The listing builds one solid part. Answer for the finished solid, in the listing's coordinates (mm). A direction names the side the tool comes from. Give positions to 0.01 mm unless a question says otherwise; leave off trailing zeros. Order: outer loops, then holes, each group sorted by start corner. A loop starts at its lowest first (then second) coordinate and runs counter-clockwise, first axis right, second up. Notation, with made-up numbers: (54.5, 72) - (62.5, 72) arc R23 cw to (62.5, 105) - close; hole circle Ø11 at (46.5, 9.25). An arc over 180 degrees is marked (long way). Write each question's results on one line, items separated by ' | '. Start each with the question number.
1. Find the intervals of material crossed by L1, parallel to X at y = 29, z = 19 (3 decimals); L2, parallel to Y at x = 2, z = 1; L3, parallel to X at y = 25, z = 20, in increasing order.
2. Flat-ended cylindrical pins translate along their axes: pin 1 (2 mm diameter, centred on x = 15.5, z = 27.5, fed in from +Y); pin 2 (10 mm diameter, centred on y = -12.5, z = -4.5, fed in from +X); pin 3 (2 mm diameter, centred on x = -3, y = 62, fed in from +Z). Find the tip coordinate at first contact, or state that the pin passes through.
3. Section A-A (y = 38.1) is taken. Give the vertices of the cut face in (x, z) (3 decimals).
4. Determine the mould class of faces 1 (the face through (-16, 3.175, -5)), 2 (the face through (22.225, 38, 9)), 3 (the face through (-25.4, 39, 18)) for opening direction X: released by +X, released by -X, zero draft, split by the parting line, or undercut.
5. Which of the six approach directions +Z, -Z, +X, -X, +Y, -Y give full straight-line access (tool end or side, diameter ignored) to faces 4 (the face through (-22.225, 38, 9)), 5 (the face through (15.92, -2.77, 14.06)), 6 (the face through (16, 3.175, -5)), 7 (the face through (15.349, -16.724, -11.197))?
from build123d import *

# Parameters (mm, degrees)
BOSS_EXTRUDE1_DEPTH                 = 25.4
SHELL1_T                            = -3.175
SKETCH4_R                           = 12.7
BOSS_EXTRUDE3_DEPTH                 = 19.05
BOSS_EXTRUDE4_DEPTH                 = 19.05
SKETCH6_R                           = 12.7
CUT_EXTRUDE2_DEPTH                  = 12.7
CUT_EXTRUDE3_START                  = 12.7
SKETCH6_2_R                         = 12.7
CUT_EXTRUDE3_DEPTH                  = 12.7
CUT_EXTRUDE4_REACH                  = 98.093
SKETCH7_R                           = 3.175
BOSS_EXTRUDE5_REACH                 = 98.093
CUT_EXTRUDE5_DEPTH                  = 12.7
BOSS_EXTRUDE6_DEPTH                 = 25.4
FILLET2_R                           = 12.7
CUT_EXTRUDE6_REACH                  = 109.812
CUT_EXTRUDE6_END_RADIUS             = 3.175
SKETCH12_R                          = 1.7526
CUT_EXTRUDE6_DIRECTION_2_REACH      = 109.812
CUT_EXTRUDE6_DIRECTION_2_END_RADIUS = 12.7
CUT_EXTRUDE7_DEPTH                  = 108.812149615


with BuildPart() as part:
    # Sketch2 → Boss-Extrude1 (new, symmetric)
    with BuildSketch(Plane(origin=(0, 0, 0), x_dir=(0, 0, -1), z_dir=(1, 0, 0))):
        with BuildLine():
            Line((0, 0), (0, 76.2))
            ThreePointArc((0, 76.2), (-38.1, 38.1), (0, 0))
        make_face()
    extrude(amount=BOSS_EXTRUDE1_DEPTH, both=True)

    # Shell1
    shell1_openings = [part.faces().sort_by_distance(p)[0] for p in [
        (0, 38.1, 0),
    ]]
    offset(amount=SHELL1_T, openings=shell1_openings)



with BuildPart() as body_2:
    # Sketch4 → Boss-Extrude3 (new, symmetric)
    with BuildSketch(Plane(origin=(0, 0, 0), x_dir=(0, 0, -1), z_dir=(1, 0, 0))):
        with Locations(Location((9.525, -9.525, 0), (0, 0, 180))):
            Circle(SKETCH4_R)
    extrude(amount=BOSS_EXTRUDE3_DEPTH, both=True)


with BuildPart() as part_1:
    add(part.part)

    add(body_2.part)  # Boss-Extrude4 merges body 2
    # Sketch5 → Boss-Extrude4 (add, symmetric)
    with BuildSketch(Plane(origin=(0, 0, 0), x_dir=(0, 0, -1), z_dir=(1, 0, 0))):
        with BuildLine():
            Line((0, 3.175), (0, 0))
            Line((0, 0), (1.124739587, 0))
            ThreePointArc((1.124739587, 0), (5.034871939, 2.354762203), (9.525, 3.175))
            Line((9.525, 3.175), (0, 3.175))
        make_face()
    extrude(amount=BOSS_EXTRUDE4_DEPTH, both=True)

    # Sketch6 → Cut-Extrude2 (cut)
    with BuildSketch(Plane(origin=(0, 0, 0), x_dir=(0, 0, -1), z_dir=(1, 0, 0))):
        with Locations((9.525, -9.525)):
            Circle(SKETCH6_R)
    extrude(amount=-CUT_EXTRUDE2_DEPTH, mode=Mode.SUBTRACT)

    # Sketch6<2> → Cut-Extrude3 (cut)
    with BuildSketch(Plane(origin=(0, 0, 0), x_dir=(0, 0, -1), z_dir=(1, 0, 0)).offset(CUT_EXTRUDE3_START)):
        with Locations((9.525, -9.525)):
            Circle(SKETCH6_2_R)
    extrude(amount=-CUT_EXTRUDE3_DEPTH, mode=Mode.SUBTRACT)

    # Cut-Extrude4: up to this face of the body (flat: up to its plane)
    cut_extrude4_end = Plane(part_1.part.faces().sort_by_distance((25.4, 38.1, 16.170142218))[0])
    # Sketch7 → Cut-Extrude4 (cut, up to the picked face)
    with BuildSketch(Plane.ZY.offset(19.05), mode=Mode.PRIVATE) as cut_extrude4_sk1:
        with Locations(Location((-9.525, -9.525, 0), (0, 0, 180))):
            Circle(SKETCH7_R)
    cut_extrude4_tool1 = split(extrude(cut_extrude4_sk1.sketch, amount=-CUT_EXTRUDE4_REACH, mode=Mode.PRIVATE), bisect_by=cut_extrude4_end, keep=Keep.BOTH, mode=Mode.PRIVATE)
    add(cut_extrude4_tool1.solids().sort_by(Axis((-19.05, -9.525, -9.525), (1, 0, 0)))[0], mode=Mode.SUBTRACT)

    # Boss-Extrude5: up to this face of the body (flat: up to its plane)
    boss_extrude5_end = Plane(part_1.part.faces().sort_by_distance((-19.05, 2.815789755, -4.7625))[0])
    # Sketch8 → Boss-Extrude5 (add, up to the picked face)
    with BuildSketch(Plane(origin=(19.05, 0, 0), x_dir=(0, 0, -1), z_dir=(1, 0, 0)), mode=Mode.PRIVATE) as boss_extrude5_sk1:
        with BuildLine():
            Line((-27.936104056, 12.192779189), (0.212965315, -18.16074027))
            Line((0.212965315, -18.16074027), (5.034871939, -21.404762203))
            Line((5.034871939, -21.404762203), (1.124739587, 0))
            Line((1.124739587, 0), (0, 3.175))
            ThreePointArc((0, 3.175), (-13.704863106, 5.9762961), (-25.211222013, 13.9308066))
            Line((-25.211222013, 13.9308066), (-27.936104056, 12.192779189))
        make_face()
    boss_extrude5_tool1 = split(extrude(boss_extrude5_sk1.sketch, amount=-BOSS_EXTRUDE5_REACH, mode=Mode.PRIVATE), bisect_by=boss_extrude5_end, keep=Keep.BOTH, mode=Mode.PRIVATE)
    add(boss_extrude5_tool1.solids().sort_by(Axis((19.05, -2.840531, 7.724646), (-1, 0, 0)))[0])

    # Sketch9 → Cut-Extrude5 (cut, symmetric)
    with BuildSketch(Plane(origin=(0, 0, 0), x_dir=(0, 0, -1), z_dir=(1, 0, 0))):
        with BuildLine():
            Line((0, 3.175), (0, 0))
            ThreePointArc((0, 0), (-15.240486985, 3.180985746), (-27.936104056, 12.192779189))
            Line((-27.936104056, 12.192779189), (0.212965315, -18.16074027))
            ThreePointArc((0.212965315, -18.16074027), (21.164671418, -14.605162328), (9.525, 3.175))
            Line((9.525, 3.175), (0, 3.175))
        make_face()
    extrude(amount=CUT_EXTRUDE5_DEPTH, both=True, mode=Mode.SUBTRACT)

    # Sketch11 → Boss-Extrude6 (add, symmetric)
    with BuildSketch(Plane(origin=(0, 0, 0), x_dir=(0, 0, -1), z_dir=(1, 0, 0))):
        Polygon((2.609832197, 76.2), (0, 76.2), (0, 73.025), align=None)
    extrude(amount=BOSS_EXTRUDE6_DEPTH, both=True)

    # Fillet2
    # the kernel refuses this fillet: 12.7 mm, written as the material it adds along each edge
    with BuildSketch(Plane(origin=(-22.225, 38.1, 0), x_dir=(0, 1, 0), z_dir=(0, 0, -1))) as fillet2_piece_1:
        with BuildLine():
            CenterArc((34.925 - FILLET2_R, FILLET2_R), FILLET2_R, 270, 90)
            Line((34.925 - FILLET2_R, 0), (34.925, 0))
            Line((34.925, 0), (34.925, FILLET2_R))
        make_face()
    revolve(axis=Axis((-22.225, 38.1, 0), (1, 0, 0)), revolution_arc=180)
    with BuildSketch(Plane(origin=(22.225, 38.1, 0), x_dir=(0, 1, 0), z_dir=(0, 0, -1))) as fillet2_piece_2:
        with BuildLine():
            CenterArc((34.925 - FILLET2_R, -FILLET2_R), FILLET2_R, 0, 90)
            Line((34.925 - FILLET2_R, 0), (34.925, 0))
            Line((34.925, 0), (34.925, -FILLET2_R))
        make_face()
    revolve(axis=Axis((22.225, 38.1, 0), (1, 0, 0)), revolution_arc=180)

    # Cut-Extrude6: up to this cylinder (the profile starts outside it)
    cut_extrude6_end = Plane(origin=(0, -9.525, -9.525), z_dir=(-1, 0, 0)) * Cylinder(CUT_EXTRUDE6_END_RADIUS, 258.724, mode=Mode.PRIVATE)
    # Sketch12 → Cut-Extrude6 (cut, up to the surface)
    with BuildSketch(Plane(origin=(0, -21.404762203, 0), x_dir=(1, 0, 0), z_dir=(0, 1, 0)), mode=Mode.PRIVATE) as cut_extrude6_sk1:
        with Locations(Location((15.875, 9.525, 0), (0, 0, 90))):
            Circle(SKETCH12_R)
    cut_extrude6_tool1 = extrude(cut_extrude6_sk1.sketch, amount=CUT_EXTRUDE6_REACH, mode=Mode.PRIVATE) - cut_extrude6_end
    add(cut_extrude6_tool1.solids().sort_by_distance((15.875, -21.404762, -9.525))[0], mode=Mode.SUBTRACT)
    # Sketch12 → Cut-Extrude6 (cut, up to the surface)
    with BuildSketch(Plane(origin=(0, -21.404762203, 0), x_dir=(1, 0, 0), z_dir=(0, 1, 0)), mode=Mode.PRIVATE) as cut_extrude6_sk2:
        with Locations(Location((-15.875, 9.525, 0), (0, 0, 90))):
            Circle(SKETCH12_R)
    cut_extrude6_tool2 = extrude(cut_extrude6_sk2.sketch, amount=CUT_EXTRUDE6_REACH, mode=Mode.PRIVATE) - cut_extrude6_end
    add(cut_extrude6_tool2.solids().sort_by_distance((-15.875, -21.404762, -9.525))[0], mode=Mode.SUBTRACT)

    # Cut-Extrude6 direction 2: up to this cylinder (the profile starts inside it)
    cut_extrude6_direction_2_end = Plane(origin=(0, -9.525, -9.525), z_dir=(-1, 0, 0)) * Cylinder(CUT_EXTRUDE6_DIRECTION_2_END_RADIUS, 277.774, mode=Mode.PRIVATE)
    # Sketch12 → Cut-Extrude6 direction 2 (cut, up to the surface)
    with BuildSketch(Plane(origin=(0, -21.404762203, 0), x_dir=(1, 0, 0), z_dir=(0, 1, 0)), mode=Mode.PRIVATE) as cut_extrude6_direction_2_sk1:
        with Locations(Location((15.875, 9.525, 0), (0, 0, 90))):
            Circle(SKETCH12_R)
    cut_extrude6_direction_2_tool1 = extrude(cut_extrude6_direction_2_sk1.sketch, amount=-CUT_EXTRUDE6_DIRECTION_2_REACH, mode=Mode.PRIVATE) & cut_extrude6_direction_2_end
    add(cut_extrude6_direction_2_tool1.solids().sort_by_distance((15.875, -21.404762, -9.525))[0], mode=Mode.SUBTRACT)
    # Sketch12 → Cut-Extrude6 direction 2 (cut, up to the surface)
    with BuildSketch(Plane(origin=(0, -21.404762203, 0), x_dir=(1, 0, 0), z_dir=(0, 1, 0)), mode=Mode.PRIVATE) as cut_extrude6_direction_2_sk2:
        with Locations(Location((-15.875, 9.525, 0), (0, 0, 90))):
            Circle(SKETCH12_R)
    cut_extrude6_direction_2_tool2 = extrude(cut_extrude6_direction_2_sk2.sketch, amount=-CUT_EXTRUDE6_DIRECTION_2_REACH, mode=Mode.PRIVATE) & cut_extrude6_direction_2_end
    add(cut_extrude6_direction_2_tool2.solids().sort_by_distance((-15.875, -21.404762, -9.525))[0], mode=Mode.SUBTRACT)

    # Sketch13 → Cut-Extrude7 (cut, through all)
    with BuildSketch(Plane(origin=(0, -21.404762203, 0), x_dir=(1, 0, 0), z_dir=(0, 1, 0))):
        Polygon((19.05, 15.875), (12.7, 15.875), (12.7, 10.397684257), (12.7, 3.175), (19.05, 3.175), align=None)
        Polygon((-19.05, 15.875), (-12.7, 15.875), (-12.7, 10.397684257), (-12.7, 3.175), (-19.05, 3.175), align=None)
    extrude(amount=-CUT_EXTRUDE7_DEPTH, mode=Mode.SUBTRACT)


solid = part_1.part
Reported:
1) L1: -25.4 to -22.225, 22.225 to 25.4 | L2: 0.01 to 3.19, 73.01 to 76.19 | L3: -25.4 to -22.11, 22.11 to 25.4
2) pin 1: y = 65.47 | pin 2: x = 19.05 | pin 3: z = 30.45
3) outline: (-25.4, 0) - (-22.225, 0) - (-22.225, 22.225) arc R12.7 cw to (-9.525, 34.925) - (9.525, 34.925) arc R12.7 cw to (22.225, 22.225) - (22.225, 0) - (25.4, 0) - (25.4, 38.1) - (-25.4, 38.1) - close
4) face 1: zero draft | face 2: undercut | face 3: released by -X
5) face 4: -Z | face 5: +Z, +X, -X, -Y | face 6: -Z, +X, -X | face 7: -Y
